Autodesk Inventor part; units mm, degrees
ref_plane "YZ Plane" through (0, 0, 0) normal (1, 0, 0) x (0, 1, 0)
ref_plane "XZ Plane" through (0, 0, 0) normal (0, 1, 0) x (-1, 0, 0)
ref_plane "XY Plane" through (0, 0, 0) normal (0, 0, 1) x (1, 0, 0)
sketch "Sketch1" plane through (0, 0, 0) normal (0, 0, 1) x (1, 0, 0)
  line L0 (-160, 166) -> (160, 166)
  line L1 (160, 166) -> (160, -166)
  line L2 (160, -166) -> (-160, -166)
  line L3 (-160, -166) -> (-160, 166)
  point P0 (0, 0)
  dimension "d0" = 320
  dimension "d1" = 332
  dimension "d2" = 160
  dimension "d3" = 166
extrude "Tykkelse" add sketch "Sketch1" along normal mid plane 6
sketch "Sketch2" plane through (0, 0, 3) normal (0, 0, 1) x (1, 0, 0)
  line L0 (-102, 98) -> (102, 98)
  line L1 (115, 85) -> (115, -107)
  line L2 (102, -120) -> (-102, -120)
  line L3 (-115, -107) -> (-115, 85)
  line L4 (160, -166) -> (160, 166)
  line L5 (-160, 166) -> (-160, -166)
  line L6 (-160, -166) -> (160, -166)
  line L7 (160, 166) -> (-160, 166)
  arc A0 (-102, 98) -> (-115, 85) centre (-102, 85) ccw
  arc A1 (115, 85) -> (102, 98) centre (102, 85) ccw
  arc A2 (102, -120) -> (115, -107) centre (102, -107) ccw
  arc A3 (-115, -107) -> (-102, -120) centre (-102, -107) ccw
  point P0 (0, 0)
  dimension "d6" = 45
  dimension "d7" = 45
  dimension "d8" = 46
  dimension "d9" = 68
  dimension "d10" = 13
  dimension "d20" = 218
  dimension "d21" = 230
extrude "Vindue" cut sketch "Sketch2" against normal up to surface (6 mm away) contours L0 A1 L1 A2 L2 A3 L3 A0
sketch "Sketch3" plane through (0, 0, -3) normal (0, 0, -1) x (-1, 0, 0)
  circle A0 centre (65, 138) radius 6
  circle A1 centre (-65, 138) radius 6
  line L0 (-65, 138) -> (65, 138) construction
  line L1 (160, 166) -> (-160, 166)
  point P0 (0, 0)
  dimension "d13" = 12
  dimension "d14" = 12
  dimension "d15" = 130
  dimension "d16" = 65
  dimension "d17" = 28
extrude "Ø12 mm huller" cut sketch "Sketch3" against normal blind 3.5
sketch "Sketch4" plane through (0, 0, 3) normal (0, 0, 1) x (1, 0, 0)
  line L0 (156, 162) -> (-156, 162) construction
  line L1 (-156, 162) -> (-156, -162) construction
  line L2 (-156, -162) -> (156, -162) construction
  line L3 (156, -162) -> (156, 162) construction
  circle A0 centre (-156, -80) radius 1.5
  circle A1 centre (-156, 0) radius 1.5
  circle A2 centre (-156, 80) radius 1.5
  circle A3 centre (-80, 162) radius 1.5
  circle A4 centre (0, 162) radius 1.5
  circle A5 centre (80, 162) radius 1.5
  circle A6 centre (156, 80) radius 1.5
  circle A7 centre (156, 0) radius 1.5
  circle A8 centre (156, -80) radius 1.5
  circle A9 centre (-80, -162) radius 1.5
  circle A10 centre (0, -162) radius 1.5
  circle A11 centre (80, -162) radius 1.5
  line L4 (-160, 166) -> (-160, -166) construction
  line L5 (-160, -166) -> (160, -166) construction
  line L6 (160, 166) -> (-160, 166) construction
  line L7 (160, -166) -> (160, 166) construction
  point P0 (0, 0)
  dimension "d22" = 3
  dimension "d23" = 3
  dimension "d24" = 3
  dimension "d25" = 3
  dimension "d26" = 3
  dimension "d27" = 3
  dimension "d28" = 3
  dimension "d29" = 3
  dimension "d30" = 3
  dimension "d31" = 3
  dimension "d32" = 3
  dimension "d33" = 3
  dimension "d34" = 4
  dimension "d35" = 4
  dimension "d36" = 4
  dimension "d37" = 4
  dimension "d38" = 240
  dimension "d39" = 160
  dimension "d40" = 80
  dimension "d41" = 80
  dimension "d42" = 160
  dimension "d43" = 240
  dimension "d44" = 86
  dimension "d45" = 166
  dimension "d46" = 246
  dimension "d47" = 246
  dimension "d48" = 166
  dimension "d49" = 86
extrude "Monteringshuller" cut sketch "Sketch4" against normal up to surface (6 mm away)
equation "\"d7\" = d6"
equation "\"d14\" = d13"
equation "\"d22\" = d23"
equation "\"d24\" = d23"
equation "\"d25\" = d23"
equation "\"d26\" = d23"
equation "\"d27\" = d23"
equation "\"d28\" = d23"
equation "\"d29\" = d23"
equation "\"d30\" = d23"
equation "\"d31\" = d23"
equation "\"d32\" = d23"
equation "\"d33\" = d23"
properties part number "Låg mk2"
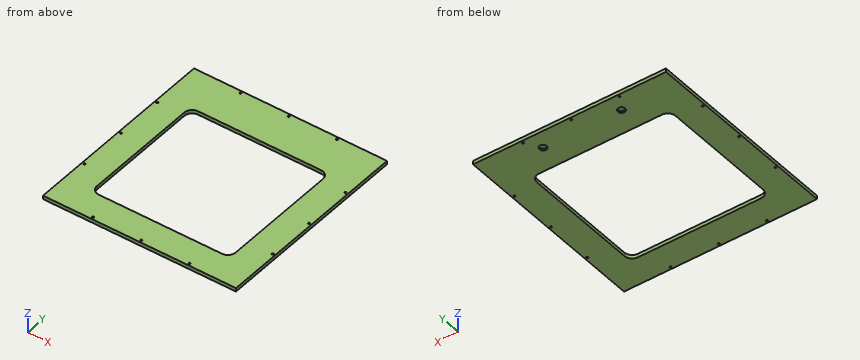
The listing builds one solid part. Answer for the finished solid, in the listing's coordinates (mm). Coordinates: 2 decimals unless noted, no trailing zeros. Write each loop counter-clockwise with the first axis right and the second up, starting at its lowest first coordinate (ties: lowest second). Pieces come first, ordered by that corner, then holes.
Q1. Find the intervals of material crossed by line 1 along Y through (x, z) = (0, 0.2); line 2 along X through (y, z) = (79.5, 0.65); line 3 along X through (y, z) = (-80, -0.4), in increasing order.
Returned:
line 1: y = -166 to -163.5, -160.5 to -120, 98 to 160.5, 163.5 to 166
line 2: x = -160 to -157.41, -154.59 to -115, 115 to 154.59, 157.41 to 160
line 3: x = -160 to -157.5, -154.5 to -115, 115 to 154.5, 157.5 to 160
Q2. Section C-C, the plane x = 20 is taken. Write down the section's boundary in (y, z).
Returned:
outline: (-166, -3) - (-120, -3) - (-120, 3) - (-166, 3) - close; (98, -3) - (166, -3) - (166, 3) - (98, 3) - close
Q3. Section B-B, the plane x = 65 is taken. Write down the section's boundary in (y, z).
Returned:
outline: (-166, -3) - (-120, -3) - (-120, 3) - (-166, 3) - close; (98, -3) - (132, -3) - (132, 0.5) - (144, 0.5) - (144, -3) - (166, -3) - (166, 3) - (98, 3) - close
Q4. Given P1, Ø6, axis at x = 66, y = 137, coming from the -Z side, flat-ended and moving along its own axis, determine where the tip first touches the part or whether it passes through.
Returned:
P1: stops at z = 0.5
Q5. Section A-A, the plane y = -96 is taken. Write down the section's boundary in (x, z), then the cut area to 3 significant figures.
Returned:
outline: (-160, -3) - (-115, -3) - (-115, 3) - (-160, 3) - close; (115, -3) - (160, -3) - (160, 3) - (115, 3) - close
area: 540 mm2
